The listing builds one solid part. Answer for the finished solid, in the listing's coordinates (mm). A direction names the side the tool comes from. Coordinates: 2 decimals unless noted, no trailing zeros. Order: outer loops, then holes, each group sorted by start corner. A loop starts at its lowest first (then second) coordinate and runs counter-clockwise, first axis right, second up. Notation, with made-up numbers: (-7, 42) -> (29, 42) arc R13 cw to (29, 56) -> close; hole circle Ø8 at (-27, 25). An arc over 180 degrees is marked (long way). Answer in a Markdown table with one row per item.
```python
from build123d import *

# Parameters (mm, degrees)
SKETCH1_W           = 20
SKETCH1_H           = 70
BOSS_EXTRUDE1_DEPTH = 3
SKETCH2_W           = 15
SKETCH2_H           = 15
BOSS_EXTRUDE2_DEPTH = 3
BOSS_EXTRUDE3_DEPTH = 3
BOSS_EXTRUDE4_DEPTH = 3
SKETCH7_R           = 5
SKETCH7_R_2         = 1.25
CUT_EXTRUDE1_DEPTH  = 4


with BuildPart() as part:
    # Sketch1 → Boss-Extrude1 (new body)
    with BuildSketch(Plane.XY):
        with Locations((-6.20477445, -5.177042891)):
            Rectangle(SKETCH1_W, SKETCH1_H)
    extrude(amount=BOSS_EXTRUDE1_DEPTH)

    # Sketch2 → Boss-Extrude2 (add)
    with BuildSketch(Plane.XY.offset(3)):
        with Locations((-23.70477445, -9.077042891)):
            Rectangle(SKETCH2_W, SKETCH2_H)
    extrude(amount=-BOSS_EXTRUDE2_DEPTH)

    # Sketch3 → Boss-Extrude3 (add)
    with BuildSketch(Plane.XY.offset(3)):
        Polygon((-31.20477445, -1.577042891), (-16.20477445, 29.822957109), (-16.20477445, -1.577042891), align=None)
        Polygon((-31.20477445, -16.577042891), (-16.20477445, -16.577042891), (-16.20477445, -40.177042891), align=None)
    extrude(amount=-BOSS_EXTRUDE3_DEPTH)

    # Sketch6 → Boss-Extrude4 (add)
    with BuildSketch(Plane.XY.offset(3)):
        Polygon((-16.20477445, -40.177042891), (-16.20477445, -45.177042891), (-21.20477445, -45.177042891), (-21.20477445, -32.310376225), align=None)
    extrude(amount=-BOSS_EXTRUDE4_DEPTH)

    # Sketch7 → Cut-Extrude1 (cut, through all)
    with BuildSketch(Plane.XY.offset(3)):
        with Locations((-23.70477445, -9.077042891)):
            Circle(SKETCH7_R)
        with Locations((-13.20477445, -36.177042891)):
            Circle(SKETCH7_R_2)
        with Locations((-6.20477445, 12.780450103)):
            Circle(SKETCH7_R)
        with Locations((-10.20477445, 25.822957109)):
            Circle(SKETCH7_R_2)
        with Locations((-2.20477445, 25.822957109)):
            Circle(SKETCH7_R_2)
        Polygon((3.79522555, -40.177042891), (3.79522555, -30.177042891), (-16.20477445, -40.177042891), align=None)
    extrude(amount=-CUT_EXTRUDE1_DEPTH, mode=Mode.SUBTRACT)


solid = part.part
```
(1) A cutting plane is placed at B-B, the plane y = -11.5. Determine the outline of the cut face in (x, z).
Check values:
| item | result |
|---|---|
| outline | (-31.2, 0) -> (-28.08, 0) -> (-28.08, 3) -> (-31.2, 3) -> close; (-19.33, 0) -> (3.8, 0) -> (3.8, 3) -> (-19.33, 3) -> close |
(2) A cutting plane is placed at A-A, the plane x = -10. Determine the outline of the cut face in (y, z), then the cut area to 3 significant figures.
Check values:
| item | result |
|---|---|
| outline | (-37.07, 0) -> (9.53, 0) -> (9.53, 3) -> (-37.07, 3) -> close; (16.04, 0) -> (24.59, 0) -> (24.59, 3) -> (16.04, 3) -> close; (27.06, 0) -> (29.82, 0) -> (29.82, 3) -> (27.06, 3) -> close |
| area | 174 mm² |
(3) A cutting plane is placed at C-C, the plane x = -23. Determine the outline of the cut face in (y, z), then the cut area to 3 significant figures.
Check values:
| item | result |
|---|---|
| outline | (-29.49, 0) -> (-14.03, 0) -> (-14.03, 3) -> (-29.49, 3) -> close; (-4.13, 0) -> (15.6, 0) -> (15.6, 3) -> (-4.13, 3) -> close |
| area | 106 mm² |
(4) Find the intervals of material crossed by line 1 along X through (y, z) = (25, 2.1); line 2 along Y through (x, z) = (-9.5, 0.25); line 3 along X through (y, z) = (-9, 2.7), in increasing order. Write a range as from..to.
Check values:
| item | result |
|---|---|
| line 1 | -18.51..-11.15, -9.26..-3.15, -1.26..3.8 |
| line 2 | -36.82..9.02, 16.54..24.79, 26.86..29.82 |
| line 3 | -31.2..-28.7, -18.71..3.8 |
(5) A cutting plane is placed at D-D, the plane z = 1.35. Determine the outline of the cut face in (x, y).
Check values:
| item | result |
|---|---|
| outline | (-31.2, -16.58) -> (-21.2, -32.31) -> (-21.2, -45.18) -> (-16.2, -45.18) -> (-16.2, -40.18) -> (3.8, -30.18) -> (3.8, 29.82) -> (-16.2, 29.82) -> (-31.2, -1.58) -> close; hole circle Ø10 at (-23.7, -9.08); hole circle Ø2.5 at (-13.2, -36.18); hole circle Ø2.5 at (-10.2, 25.82); hole circle Ø10 at (-6.2, 12.78); hole circle Ø2.5 at (-2.2, 25.82) |
(6) Which of the six approach directions +Z, -Z, +X, -X, +Y, -Y give full straight-line access (tool end or side, diameter ignored) to faces 1 (the flat face through (-21.205, -39, 2)), 2 (the flat face through (-16.205, -43, 2)), 3 (the flat face through (3.795, -1, 1))?
Check values:
| item | result |
|---|---|
| face 1 | +Z, -Z, -X, -Y |
| face 2 | +Z, -Z, +X, -Y |
| face 3 | +Z, -Z, +X, +Y, -Y |
(7) For a pull along Y with two mould halves and no side action, classify faces 4 (the flat face through (-23.81, 13.9, 1.52)), 5 (the cylindrical face through (-6.856, 17.738, 1.521)), 6 (the flat face through (-13, -7, 3)) as released by +Y, released by -Y, zero draft, split by the parting line, or undercut.
Check values:
| item | result |
|---|---|
| face 4 | released by +Y |
| face 5 | undercut |
| face 6 | zero draft |
